The drawing under review shows one solid part. Ordinate dimensions are in mm from its lowest x, y, z. Give positions to 0.01 mm unless a question says otherwise; leave off trailing zeros. Order: outer loops, then holes, each group sorted by start corner. A loop starts at its lowest first (then second) coordinate and runs counter-clockwise, first axis right, second up. Notation, with made-up numbers: (50, 60) -> (64, 60) arc R29 cw to (64, 83) -> close; hole circle Ø11 at (7.25, 83.5). An arc over 180 degrees is marked (long way). Use a Markdown table: item, result. Add a question column.
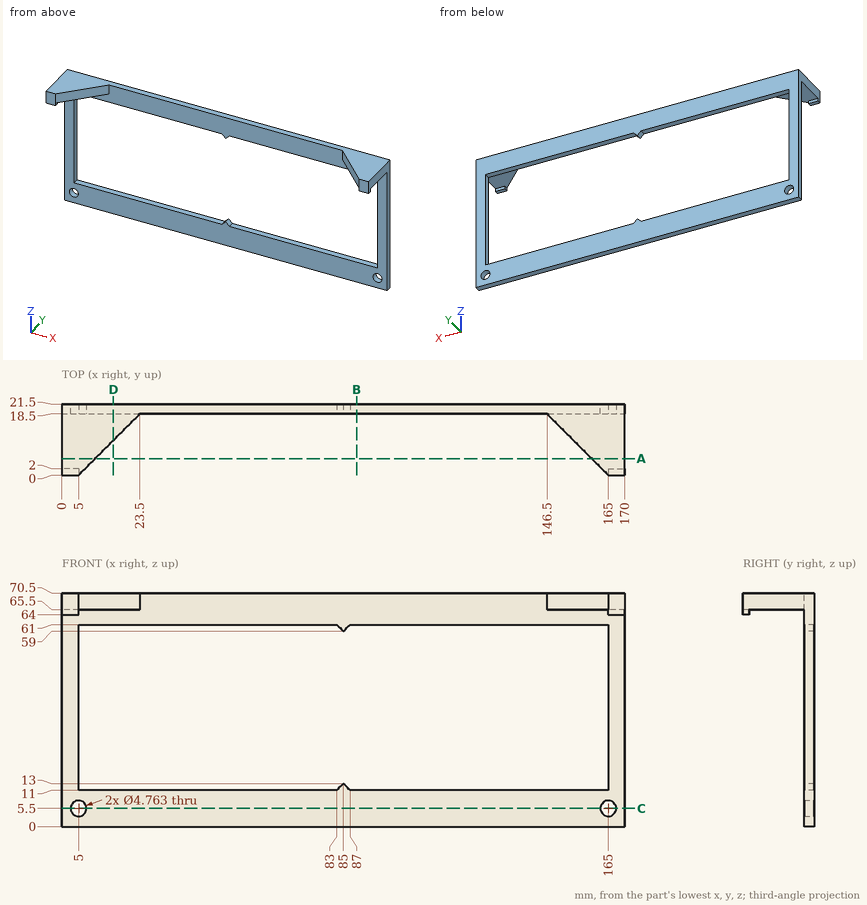
1) Add section C-C (z = 5.5). Give the boundary of the cut face in (x, y).
2) For L1, parallel to X at y = 19.5, z = 55.5; L2, parallel to Y at x = 80, z = 5, list the stretches that pass through material, from the lowest coordinate up. Write a range as [from, to].
3) Insertion check: pin 1 (4 mm diameter, centred on x = 54, y = 16, fed in from -Z); pin 2 (1.2 mm diameter, centred on y = 0.5, z = 64.5, fed in from -X); pin 3 (5.5 mm diameter, centred on x = 13.5, y = 11.5, fed in from -Z); pin 4 (1.6 mm diameter, centred on x = 168, y = 1, fed in from -Z). Each pin has a flat end and moves straight along its axis. Give the tip position at first contact, or say it passes through.
4) Add section D-D (x = 15.5). Give the boundary of the cut face in (y, z).
5) Add section B-B (x = 89). Give the boundary of the cut face in (y, z).
6) Add section A-A (y = 5). Give the boundary of the cut face in (x, z), then the cut area to 3 significant figures.
Worked answers:
| question | item | result |
|---|---|---|
| 1 | outline | (0, 18.5) -> (2.62, 18.5) -> (2.62, 21.5) -> (0, 21.5) -> close; (7.38, 18.5) -> (162.62, 18.5) -> (162.62, 21.5) -> (7.38, 21.5) -> close; (167.38, 18.5) -> (170, 18.5) -> (170, 21.5) -> (167.38, 21.5) -> close |
| 2 | L1 | [0, 5], [165, 170] |
| 2 | L2 | [18.5, 21.5] |
| 3 | pin 1 | through |
| 3 | pin 2 | x = 0 |
| 3 | pin 3 | z = 65.5 |
| 3 | pin 4 | z = 64 |
| 4 | outline | (10.5, 65.5) -> (18.5, 65.5) -> (18.5, 61) -> (21.5, 61) -> (21.5, 70.5) -> (10.5, 70.5) -> close; (18.5, 0) -> (21.5, 0) -> (21.5, 11) -> (18.5, 11) -> close |
| 5 | outline | (18.5, 0) -> (21.5, 0) -> (21.5, 11) -> (18.5, 11) -> close; (18.5, 61) -> (21.5, 61) -> (21.5, 70.5) -> (18.5, 70.5) -> close |
| 6 | outline | (0, 65.5) -> (10, 65.5) -> (10, 70.5) -> (0, 70.5) -> close; (160, 65.5) -> (170, 65.5) -> (170, 70.5) -> (160, 70.5) -> close |
| 6 | area | 100 mm^2 |
